Can you work these out from the drawing? Everything is in mm from the part's minimum corner. Coordinates: 2 decimals unless noted, no trailing zeros. Loops run counter-clockwise (first coordinate to the right, second up) from the corner with the lowest first, then second, coordinate; pieces in that order, holes last. Notation, with made-up numbers: M 42,75.25 L 55,75.25 A5 cw 55,81.25 Z; hole C 31.25,-5 d1. An arc over 180 degrees is marked long. Use CSV: the item, a comma, the result in double quotes. Start each with the question number.
Q1. If we section it at C-C (y = 117): Please give me the cut outline in (x, z), and give its area (3 significant figures).
Q2. Please list where these lines run through material, in increasing order: probe 1 along X at (y, z) = (101, 0.6); probe 2 along Y at (x, z) = (73, 2.5). Write a range as [from, to].
Q3. For pin 1 Ø1.5 at (x, z) = (80.5, 2) entering from -Y, with a flat end and sliding along its axis, tell me the tip position at first contact or that it passes through.
Q4. If we section it at A-A (z = 1): Please give me the cut outline in (x, y).
Q5. If we section it at B-B (x = 81.5): Please give me the cut outline in (y, z).
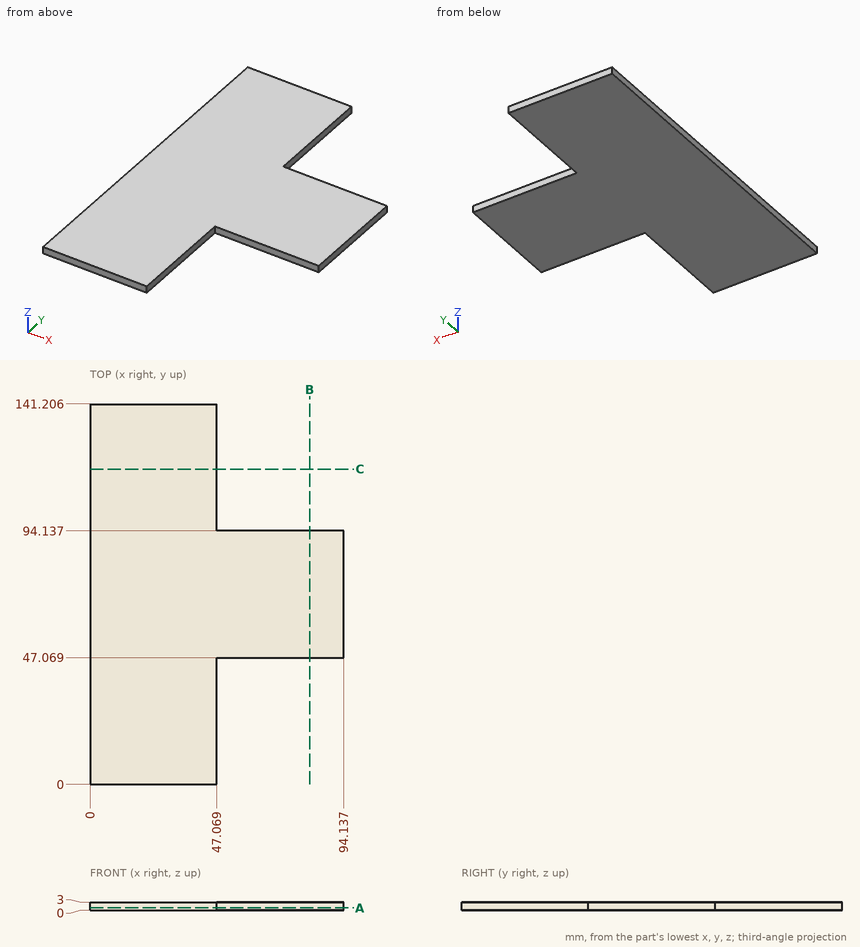
Results below:
1,outline,"M 0,0 L 47.07,0 L 47.07,3 L 0,3 Z"
1,area,"141 mm^2"
2,probe 1,"[0, 47.07]"
2,probe 2,"[47.07, 94.14]"
3,pin 1,"y = 47.07"
4,outline,"M 0,0 L 47.07,0 L 47.07,47.07 L 94.14,47.07 L 94.14,94.14 L 47.07,94.14 L 47.07,141.21 L 0,141.21 Z"
5,outline,"M 47.07,0 L 94.14,0 L 94.14,3 L 47.07,3 Z"
